Autodesk Inventor part; units mm, degrees
ref_plane "YZ Plane" through (0, 0, 0) normal (1, 0, 0) x (0, 1, 0)
ref_plane "XZ Plane" through (0, 0, 0) normal (0, 1, 0) x (-1, 0, 0)
ref_plane "XY Plane" through (0, 0, 0) normal (0, 0, 1) x (1, 0, 0)
sketch "Sketch1" plane through (0, 0, 0) normal (0, 1, 0) x (-1, 0, 0)
  line L0 (-25, 12.5) -> (25, 12.5)
  line L1 (25, 12.5) -> (25, -12.5)
  line L2 (25, -12.5) -> (-25, -12.5)
  line L3 (-25, -12.5) -> (-25, 12.5)
  line L4 (-25, 12.5) -> (25, -12.5) construction
  line L5 (25, 12.5) -> (-25, -12.5) construction
  line L6 (27, 14) -> (27, -14)
  line L7 (-25, 12.5) -> (-25, 14)
  line L8 (-25, 14) -> (27, 14)
  line L9 (27, -14) -> (-25, -14)
  line L10 (-25, -14) -> (-25, -12.5)
  line L11 (25, 12.5) -> (27, 12.5)
  line L12 (25, -12.5) -> (27, -12.5)
  line L13 (-25, -14) -> (27, -14)
  line L14 (27, -14) -> (27, -22)
  line L15 (27, -22) -> (-25, -22)
  line L16 (-25, -22) -> (-25, -14)
  line L17 (27, 0) -> (-25, 0)
  line L18 (-25, 14) -> (27, 14)
  line L19 (27, 14) -> (27, 22)
  line L20 (27, 22) -> (-25, 22)
  line L21 (-25, 22) -> (-25, 14)
  point P0 (0, 0)
  point P1 (27, 14)
  dimension "d0" = 25
  dimension "d1" = 50
  dimension "d2" = 2
  dimension "d3" = 1.5
  dimension "d4" = 1.5
  dimension "d60" = 8
extrude "Extrusion1" add sketch "Sketch1" against normal blind 2 contours L7 L8 L6 L11 L0 | L0 L1 L17 L3 | L11 L6 L17 L1 | L17 L1 L2 L3 | L17 L6 L12 L1 | L2 L12 L6 L9 L10
extrude "Extrusion2" add sketch "Sketch1" along normal blind 18.8 contours L7 L8 L6 L11 L0 | L2 L12 L6 L9 L10
sketch "Sketch2" plane through (-27, 0, -12.5) normal (0, 0, 1) x (1, 0, 0)
  line L0 (0, 18.8) -> (0, 20)
  line L1 (0, 0) -> (0, 18.8)
  line L2 (0, 18.8) -> (2, 18.8)
  line L3 (0, 18.8) -> (52, 18.8)
  line L4 (2, 18.8) -> (2, 11.5)
  line L5 (52, 0) -> (0, 0)
  line L6 (2, 11.5) -> (0, 11.5)
  line L7 (0, -2) -> (0, 18.8)
  point P0 (27, 0)
  dimension "d13" = 11.5
  dimension "d14" = 20
  dimension "d15" = 2
extrude "Extrusion3" add sketch "Sketch2" along normal up to surface (25 mm away)
sketch "Sketch4" plane through (-27, -2, 14) normal (0, 0, 1) x (1, 0, 0)
  circle A0 centre (62.8, 17) radius 2.575
  circle A1 centre (62.8, 17) radius 3.1
  circle A2 centre (62.8, 17) radius 3.8
  line L0 (52, 2) -> (52, 20.8)
  line L1 (52, 12) -> (66.6, 12)
  line L2 (66.6, 12) -> (66.6, 20.8)
  line L3 (66.6, 20.8) -> (52, 20.8)
  point P0 (27, 2)
  dimension "d31" = 5.15
  dimension "d32" = 6.2
  dimension "d33" = 0.7
  dimension "d34" = 10
  dimension "d35" = 15
  dimension "d61" = 14.6
extrude "Extrusion4" add sketch "Sketch4" against normal up to surface (28 mm away) contours A1 | A2 | L2 L1 L0 L3 A2 | A2 L3 L2
sketch "Sketch5" plane through (25, -2, 14) normal (1, 0, 0) x (0, 0, -1)
  line L0 (0, 0) -> (0, 12)
  line L1 (0, 2) -> (28, 2)
  line L2 (28, 0) -> (28, 12)
  line L3 (1.5, 2) -> (26.5, 2)
  line L4 (28, 12) -> (26.5, 12)
  line L5 (26.5, 2) -> (26.5, 12)
  line L6 (1.5, 12) -> (1.5, 2)
  line L7 (26.5, 12) -> (1.5, 12)
  line L8 (26.5, 12) -> (26.5, 20.8)
  line L9 (26.5, 20.8) -> (28, 20.8)
  line L10 (28, 20.8) -> (28, 12)
  line L11 (28, 12) -> (28, 0)
  line L12 (28, 0) -> (0, 0)
  line L13 (0, 0) -> (0, 12)
  line L14 (0, 12) -> (0, 20.8)
  line L15 (0, 20.8) -> (1.5, 20.8)
  line L16 (1.5, 20.8) -> (1.5, 12)
  line L17 (1.5, 12) -> (0, 12)
  line L18 (1.5, 20.8) -> (26.5, 20.8)
  line L19 (1.5, 2) -> (26.5, 2)
  point P0 (14, 2)
extrude "Extrusion6" add sketch "Sketch5" along normal up to surface (14.6 mm away) contours L0 L1 L2 L12
extrude "Extrusion8" add sketch "Sketch5" along normal blind 4 contours L0 L17 L6 L1 | L1 L5 L4 L2
extrude "Extrusion9" add sketch "Sketch4" along normal blind 1 contours A2
extrude "Extrusion10" add sketch "Sketch4" along normal blind 0.1 contours A1
sketch "Sketch7" plane through (-27, -2, -14) normal (0, 0, -1) x (-1, 0, 0)
  circle A0 centre (-62.8, 17) radius 3.8
  circle A1 centre (-62.8, 17) radius 3.1
  circle A2 centre (-62.8, 17) radius 3.1
  circle A3 centre (-62.8, 17) radius 2.575
  point P0 (-27, 2)
extrude "Extrusion11" add sketch "Sketch7" along normal blind 0.1 contours A1
extrude "Extrusion12" add sketch "Sketch7" along normal blind 1 contours A0
extrude "Extrusion13" add sketch "Sketch1" against normal up to surface (2 mm away) contours L21 L20 L19 L8 | L9 L14 L15 L16
sketch "Sketch8" plane through (25, 0, 22) normal (1, 0, 0) x (0, 0, -1)
  line L0 (0, -2) -> (8, -2)
  line L1 (8, 0) -> (8, -2)
  line L2 (0, 0) -> (8, 0)
  line L3 (0, 0) -> (0, -2)
  line L4 (36, -2) -> (44, -2)
  line L5 (44, 0) -> (44, -2)
  line L6 (36, 0) -> (44, 0)
  line L7 (36, -2) -> (36, 0)
  point P0 (22, 0)
extrude "Extrusion14" add sketch "Sketch8" along normal up to surface (14.6 mm away)
equation "\"d4\" = d3"
equation "\"d15\" = d2"
properties part number "chaimber"
Verification items for the finished model (mm, model axes). A direction names the side the tool comes from. Round coordinates to 2 decimals unless told otherwise and drop trailing zeros. Write each loop counter-clockwise with the first axis right and the second up, starting at its lowest first coordinate (ties: lowest second). Pieces come first, ordered by that corner, then holes. Notation, with made-up numbers: (66.25, -4.5) - (87.25, -4.5) arc R34 cw to (87.25, 25.5) - close; hole circle Ø11 at (84.5, 31). An arc over 180 degrees is marked (long way). Answer as a JSON object with one key per item and string values. Group by question number.
Q1. Section check B-B, the plane x = 16. Enter the section's corners in (y, z), plus the area to 3 significant figures.
Q2. Section check C-C, the plane z = 16. Enter the section's corners in (x, y), plus the area to 3 significant figures.
Q3. Section check A-A, the plane z = 0. Enter the section's corners in (x, y) (3 decimals).
Q4. Go/stop test with flat-tipped pins: pin 1 Ø6.5 at (x, y) = (35.8, 15) entering from +Z; pin 2 Ø22 at (x, z) = (11.5, 6.5) entering from +Y; pin 3 Ø4 at (x, y) = (37, 17.5) entering from -Z; pin 4 Ø1 at (x, y) = (-6, 7.5) entering from -Z. Record where each tip stops, or that it passes through.
Q5. Tool access check on faces 1 (the flat face through (39, 18, -14)), 2 (the cylindrical face through (38.664, 16.187, 14.544)), 3 (the flat face through (29, 5, -13)). Record the directions out of +Z, -Z, +X, -X, +Y, -Y that give a thin tool (end or side, any length) a straight path to the whole face; none if there is none.
Q6. Mould release check, pull along Y, two halves, no side actions. Record for faces 4 (the flat face through (26, 18.8, 0)), 5 (the flat face through (32, 10, 0)), 6 (the flat face through (39.6, 14, 0)), 7 (the cylindrical face through (39.425, 13.859, 14.493)): released by +Y, released by -Y, zero draft, split by the parting line, or undercut.
Q7. Thickness scan on line 1 (Y direction, x = 35.8, z = 14.45); line 2 (Z direction, x = 22, y = 15.25); line 3 (X direction, y = 13, z = 3). Record the ranges inside material, lowest first.
Found:
{
 "1": {"outline": "(-2, -22) - (0, -22) - (0, -14) - (18.8, -14) - (18.8, -12.5) - (0, -12.5) - (0, 12.5) - (18.8, 12.5) - (18.8, 14) - (0, 14) - (0, 22) - (-2, 22) - close", "area": "144 mm^2"},
 "2": {"outline": "(-27, -2) - (39.6, -2) - (39.6, 0) - (-27, 0) - close", "area": "133 mm^2"},
 "3": {"outline": "(-27, -2) - (39.6, -2) - (39.6, 0) - (-27, 0) - close; (-27, 11.5) - (-25, 11.5) - (-25, 18.8) - (-27, 18.8) - close; (25, 10) - (39.6, 10) - (39.6, 18.8) - (25, 18.8) - close; hole circle Ø5.15 at (35.8, 15)"},
 "4": {"pin 1": "stops at z = 15", "pin 2": "stops at y = 18.8", "pin 3": "stops at z = -15", "pin 4": "stops at z = -14"},
 "5": {"face 1": "-Z, +X, +Y", "face 2": "+Z", "face 3": "+Z, -Z, +X"},
 "6": {"face 4": "released by +Y", "face 5": "undercut", "face 6": "zero draft", "face 7": "undercut"},
 "7": {"line 1": "y = -2 to 0, 11.2 to 11.9, 18.1 to 18.8", "line 2": "z = -14 to -12.5, 12.5 to 14", "line 3": "x = -27 to -25, 25 to 34.18, 37.42 to 39.6"}
}
